from build123d import *

# Parameters (mm, degrees)
SKETCH1_W           = 63.5
SKETCH1_H           = 63.5
BOSS_EXTRUDE1_DEPTH = 1.27
SKETCH2_R           = 1.905
CUT_EXTRUDE1_DEPTH  = 1.27
SKETCH3_W           = 44.45
SKETCH3_H           = 19.05
CUT_EXTRUDE2_DEPTH  = 1.27
SKETCH4_R           = 0.73025
BOSS_EXTRUDE2_DEPTH = 3.81
CUT_EXTRUDE3_REACH  = 5.81
SKETCH5_W           = 26.162
SKETCH5_H           = 19.685
SKETCH6_R           = 0.73025
CUT_EXTRUDE4_DEPTH  = 4.81


with BuildPart() as part:
    # Sketch1 → Boss-Extrude1 (new body)
    with BuildSketch(Plane(origin=(0, 0, 0), x_dir=(1, 0, 0), z_dir=(0, 1, 0))):
        Rectangle(SKETCH1_W, SKETCH1_H)
    extrude(amount=BOSS_EXTRUDE1_DEPTH)

    # Sketch2 → Cut-Extrude1 (cut)
    with BuildSketch(Plane(origin=(0, 1.27, 0), x_dir=(1, 0, 0), z_dir=(0, 1, 0))):
        with Locations((27.0129, 6.985)):
            Circle(SKETCH2_R)
        with Locations((26.162, 26.67)):
            Circle(SKETCH2_R)
        with Locations((-27.0129, 6.985)):
            Circle(SKETCH2_R)
        with Locations((-26.162, 26.67)):
            Circle(SKETCH2_R)
    extrude(amount=-CUT_EXTRUDE1_DEPTH, mode=Mode.SUBTRACT)

    # Sketch3 → Cut-Extrude2 (cut)
    with BuildSketch(Plane(origin=(0, 1.27, 0), x_dir=(1, 0, 0), z_dir=(0, 1, 0))):
        with Locations((0, 15.875)):
            Rectangle(SKETCH3_W, SKETCH3_H)
    extrude(amount=-CUT_EXTRUDE2_DEPTH, mode=Mode.SUBTRACT)

    # Sketch4 → Boss-Extrude2 (add)
    with BuildSketch(Plane(origin=(0, 1.27, 0), x_dir=(1, 0, 0), z_dir=(0, 1, 0))):
        with Locations((-15.748, -7.3025)):
            Circle(SKETCH4_R)
        with Locations((15.748, -19.3167)):
            Circle(SKETCH4_R)
    extrude(amount=-BOSS_EXTRUDE2_DEPTH)

    # Sketch5 → Cut-Extrude3 (cut, up to next)
    with BuildSketch(Plane(origin=(0, 1.27, 0), x_dir=(1, 0, 0), z_dir=(0, 1, 0)), mode=Mode.PRIVATE) as cut_extrude3_sk1:
        with Locations((0, -15.875)):
            Rectangle(SKETCH5_W, SKETCH5_H)
    cut_extrude3_tool1 = extrude(cut_extrude3_sk1.sketch, amount=-CUT_EXTRUDE3_REACH, mode=Mode.PRIVATE) & part.part
    add(cut_extrude3_tool1.solids().sort_by_distance((0, 1.27, 15.875))[0], mode=Mode.SUBTRACT)

    # Sketch6 → Cut-Extrude4 (cut, through all)
    with BuildSketch(Plane.XZ.offset(2.54)):
        with Locations((15.748, 19.3167)):
            Circle(SKETCH6_R)
        with Locations((-15.748, 7.3025)):
            Circle(SKETCH6_R)
    extrude(amount=-CUT_EXTRUDE4_DEPTH, mode=Mode.SUBTRACT)


solid = part.part
Can you work these out from the model? Positions are in its coordinate system, mm. Round coordinates to 2 decimals unless told otherwise and drop trailing zeros. Order: outer loops, then holes, each group sorted by start corner. A loop starts at its lowest first (then second) coordinate and runs counter-clockwise, first axis right, second up. Notation, with made-up numbers: M 83,61 L 108,61 A28 cw 108,80 Z; hole C 76.25,31.5 d4. An arc over 180 degrees is marked long. Use a Markdown table: item, result.
1) Imagine slicing it at B-B (x = 0). List the corners of the cut face in (y, z) for me, then the cut area to 3 significant figures.
Geometry says:
| item | result |
|---|---|
| outline | M 0,-31.75 L 1.27,-31.75 L 1.27,-25.4 L 0,-25.4 Z; M 0,-6.35 L 1.27,-6.35 L 1.27,6.03 L 0,6.03 Z; M 0,25.72 L 1.27,25.72 L 1.27,31.75 L 0,31.75 Z |
| area | 31.5 mm² |
2) Imagine slicing it at A-A (z = -19). List the corners of the cut face in (x, y) for me (3 decimals), then the cut area to 3 significant figures.
Geometry says:
| item | result |
|---|---|
| outline | M -31.75,0 L -22.225,0 L -22.225,1.27 L -31.75,1.27 Z; M 22.225,0 L 31.75,0 L 31.75,1.27 L 22.225,1.27 Z |
| area | 24.2 mm² |
3) If we mould it in two halves opening along X, with no side actions, what happens to faces 1 (the face through (16, 1, 20)), 2 (the face through (27.92, 0.64, -25.94)), 3 (the face through (0, 1.27, 0))? For each: +X half, -X half, draft (parallel to the pull), parting line (faces both ways), or undercut.
Geometry says:
| item | result |
|---|---|
| face 1 | undercut |
| face 2 | undercut |
| face 3 | draft |
4) I'm going to push a flat-ended pin straight in: P1, Ø2.5, axis at x = 27.01, z = -6.98, coming from the +Y side. Where does the tip first touch, or does it pass through?
Geometry says:
| item | result |
|---|---|
| P1 | passes through |
5) Imagine slicing it at D-D (z = 13.5). List the corners of the cut face in (x, y) for me.
Geometry says:
| item | result |
|---|---|
| outline | M -31.75,0 L -13.08,0 L -13.08,1.27 L -31.75,1.27 Z; M 13.08,0 L 31.75,0 L 31.75,1.27 L 13.08,1.27 Z |
6) If I drill on line 1 along X through (y, z) = (0.6, -26.67); line 2 along Z through (x, y) = (-5, 0.9); line 3 along Z through (x, y) = (-13.5, 0.6), over which ranges is the centre line in solid material (lowest first)?
Geometry says:
| item | result |
|---|---|
| line 1 | x = -31.75 to -28.07, -24.26 to 24.26, 28.07 to 31.75 |
| line 2 | z = -31.75 to -25.4, -6.35 to 6.03, 25.72 to 31.75 |
| line 3 | z = -31.75 to -25.4, -6.35 to 31.75 |
7) Imagine slicing it at C-C (z = -26.67). List the corners of the cut face in (x, y) for me.
Geometry says:
| item | result |
|---|---|
| outline | M -31.75,0 L -28.07,0 L -28.07,1.27 L -31.75,1.27 Z; M -24.26,0 L 24.26,0 L 24.26,1.27 L -24.26,1.27 Z; M 28.07,0 L 31.75,0 L 31.75,1.27 L 28.07,1.27 Z |
